Drawing for the job (mm, zero at the part's lowest x, y, z). Round coordinates to 2 decimals unless told otherwise and drop trailing zeros. Loops run counter-clockwise (first coordinate to the right, second up) from the corner with the lowest first, then second, coordinate; pieces in that order, holes last. Notation, with made-up numbers: (-12, 26) -> (31, 26) arc R17 cw to (31, 32) -> close; hole circle Ø1 at (-1.5, 75.5). An arc over 180 degrees is marked (long way). Put each result on its own line as item: value. Start each with the question number.
Item 1: Drill centre lines: probe 1 along X at (y, z) = (4.25, 112); probe 2 along Z at (x, y) = (47, 4.5); probe 3 along Z at (x, y) = (143, 3.75). Where is each one in solid material? Low to high. Write a range as [from, to].
Item 2: Cut at A-A, the plane z = 87.5. List the corners of the cut face in (x, y).
Item 3: Cut at C-C, the plane z = 116. List the corners of the cut face in (x, y), plus the area to 3 significant figures.
Item 4: Cut at B-B, the plane x = 61.5. List the corners of the cut face in (y, z), plus the area to 3 significant figures.
Item 5: Cut at D-D, the plane y = 4.25. List the corners of the cut face in (x, z).
Item 6: Flat gauge pins, fed straight in: pin 1 Ø1.9 at (y, z) = (4.5, 123.5) entering from +X; pin 2 Ø1.9 at (x, y) = (10.5, 2) entering from +Z; pin 3 Ø3 at (x, y) = (17, 2) entering from -Z. Where does each tip first touch, or does it go through?
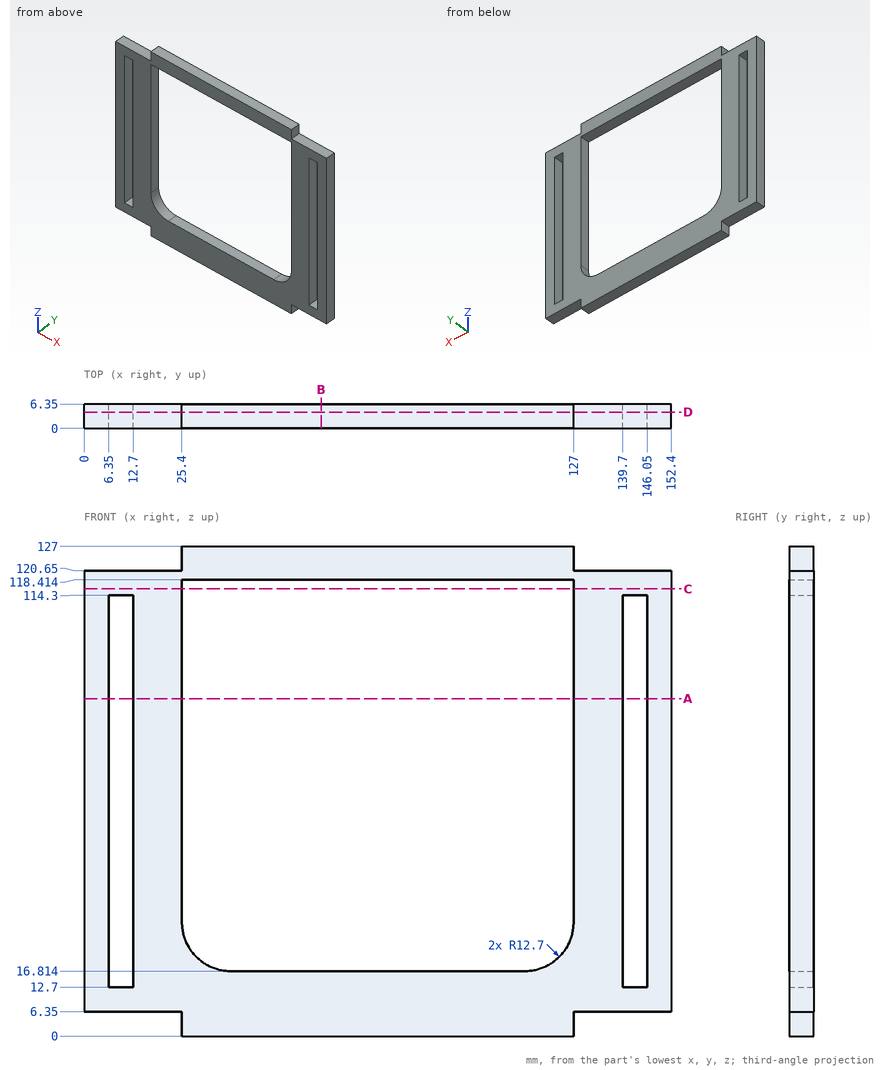
Reply:
1. probe 1: x = [0, 6.35], [12.7, 25.4], [127, 139.7], [146.05, 152.4]
1. probe 2: z = [0, 16.81], [118.41, 127]
1. probe 3: z = [6.35, 12.7], [114.3, 120.65]
2. outline: (0, 0) -> (6.35, 0) -> (6.35, 6.35) -> (0, 6.35) -> close; (12.7, 0) -> (25.4, 0) -> (25.4, 6.35) -> (12.7, 6.35) -> close; (127, 0) -> (139.7, 0) -> (139.7, 6.35) -> (127, 6.35) -> close; (146.05, 0) -> (152.4, 0) -> (152.4, 6.35) -> (146.05, 6.35) -> close
3. outline: (0, 0) -> (25.4, 0) -> (25.4, 6.35) -> (0, 6.35) -> close; (127, 0) -> (152.4, 0) -> (152.4, 6.35) -> (127, 6.35) -> close
3. area: 323 mm^2
4. outline: (0, 0) -> (6.35, 0) -> (6.35, 16.81) -> (0, 16.81) -> close; (0, 118.41) -> (6.35, 118.41) -> (6.35, 127) -> (0, 127) -> close
4. area: 161 mm^2
5. outline: (0, 6.35) -> (25.4, 6.35) -> (25.4, 0) -> (127, 0) -> (127, 6.35) -> (152.4, 6.35) -> (152.4, 120.65) -> (127, 120.65) -> (127, 127) -> (25.4, 127) -> (25.4, 120.65) -> (0, 120.65) -> close; hole (6.35, 12.7) -> (12.7, 12.7) -> (12.7, 114.3) -> (6.35, 114.3) -> close; hole (25.4, 29.51) arc R12.7 ccw to (38.1, 16.81) -> (114.3, 16.81) arc R12.7 ccw to (127, 29.51) -> (127, 118.41) -> (25.4, 118.41) -> close; hole (139.7, 12.7) -> (146.05, 12.7) -> (146.05, 114.3) -> (139.7, 114.3) -> close
6. pin 1: stops at x = 127
6. pin 2: stops at z = 120.65
6. pin 3: stops at z = 6.35
